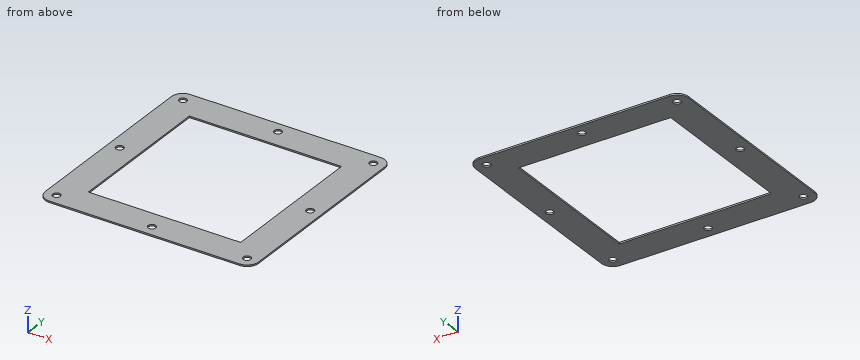
from build123d import *

# Parameters (mm, degrees)
SKETCH2_R           = 5
SKETCH2_R_2         = 4
BOSS_EXTRUDE1_DEPTH = 2
SKETCH3_W           = 200
SKETCH3_H           = 200
CUT_EXTRUDE1_DEPTH  = 10


with BuildPart() as part:
    # Sketch2 → Boss-Extrude1 (new body)
    with BuildSketch(Plane.XY):
        with BuildLine():
            Line((-125, 140), (125, 140))
            ThreePointArc((125, 140), (135.606601718, 135.606601718), (140, 125))
            Line((140, 125), (140, -125))
            ThreePointArc((140, -125), (135.606601718, -135.606601718), (125, -140))
            Line((125, -140), (-125, -140))
            ThreePointArc((-125, -140), (-135.606601718, -135.606601718), (-140, -125))
            Line((-140, -125), (-140, 125))
            ThreePointArc((-140, 125), (-135.606601718, 135.606601718), (-125, 140))
        make_face()
        with Locations((-125, 125)):
            Circle(SKETCH2_R, mode=Mode.SUBTRACT)
        with Locations((0, 125)):
            Circle(SKETCH2_R, mode=Mode.SUBTRACT)
        with Locations((125, 125)):
            Circle(SKETCH2_R, mode=Mode.SUBTRACT)
        Circle(SKETCH2_R_2, mode=Mode.SUBTRACT)
        with Locations((125, 0)):
            Circle(SKETCH2_R, mode=Mode.SUBTRACT)
        with Locations((-125, 0)):
            Circle(SKETCH2_R, mode=Mode.SUBTRACT)
        with Locations((-125, -125)):
            Circle(SKETCH2_R, mode=Mode.SUBTRACT)
        with Locations((0, -125)):
            Circle(SKETCH2_R, mode=Mode.SUBTRACT)
        with Locations((125, -125)):
            Circle(SKETCH2_R, mode=Mode.SUBTRACT)
    extrude(amount=BOSS_EXTRUDE1_DEPTH)

    # Sketch3 → Cut-Extrude1 (cut)
    with BuildSketch(Plane.XY.offset(2)):
        Rectangle(SKETCH3_W, SKETCH3_H)
    extrude(amount=-CUT_EXTRUDE1_DEPTH, mode=Mode.SUBTRACT)


solid = part.part
For this review, take the finished solid that the model builds, in its own axes (mm). Give positions to 0.01 mm unless a question says otherwise; leave off trailing zeros. Loops run counter-clockwise (first coordinate to the right, second up) from the corner with the lowest first, then second, coordinate; pieces in that order, holes last. Notation, with made-up numbers: M 51.5,32 L 77.5,32 A23 cw 77.5,64 Z; hole C 39.25,47.5 d3. An arc over 180 degrees is marked long. Put each result on its own line as item: value. Start each with the question number.
(1) Add section A-A, the plane y = 0. Write out the cut boundary in (x, z).
(2) Add section C-C, the plane z = 1.5. Give the number of separate pieces and of enclosed holes in the cut face, then the cut area to 3 significant figures.
(3) Add section D-D, the plane y = -84. Write out the cut boundary in (x, z), then the cut area to 3 significant figures.
(4) Wall thickness on L1, parallel to Y at x = 125, z = 0.4; L2, parallel to Y at x = 39.5, z = 0.6: over which ranges is each line inside the solid? List them lowest first.
Result:
1. outline: M -140,0 L -130,0 L -130,2 L -140,2 Z; M -120,0 L -100,0 L -100,2 L -120,2 Z; M 100,0 L 120,0 L 120,2 L 100,2 Z; M 130,0 L 140,0 L 140,2 L 130,2 Z
2. separate pieces: 1
2. enclosed holes: 9
2. area: 37,600 mm^2
3. outline: M -140,0 L -100,0 L -100,2 L -140,2 Z; M 100,0 L 140,0 L 140,2 L 100,2 Z
3. area: 160 mm^2
4. L1: y = -140 to -130, -120 to -5, 5 to 120, 130 to 140
4. L2: y = -140 to -100, 100 to 140
